```python
from build123d import *

# Parameters (mm, degrees)
F0_R      = 8.001
F0_R_2    = 5.08
F1_DEPTH  = 69.342
F2_R      = 8.001
F2_R_2    = 5.08
F3_ANGLE  = 90
F4_R      = 8.001
F4_R_2    = 5.08
F5_DEPTH  = 76.2
F6_R      = 8.001
F6_R_2    = 5.08
F7_ANGLE  = 30
F8_R      = 8.001
F8_R_2    = 5.08
F9_DEPTH  = 15.24
F10_R     = 8.001
F10_R_2   = 5.08
F11_ANGLE = 30
F12_R     = 8.001
F12_R_2   = 5.08
F13_DEPTH = 50.8


with BuildPart() as f1:
    # F0 (on Front) → F1 (new body)
    with BuildSketch(Plane.XZ):
        Circle(F0_R)
        Circle(F0_R_2, mode=Mode.SUBTRACT)
    extrude(amount=F1_DEPTH)

    # F2 (on face) → F3 (revolve)
    with BuildSketch(Plane.XZ.offset(69.342)):
        Circle(F2_R)
        Circle(F2_R_2, mode=Mode.SUBTRACT)
    revolve(axis=Axis((19.05, -69.342, 0.0863848254), (0, 0, 1)), revolution_arc=F3_ANGLE)

    # F4 (on face) → F5 (join)
    with BuildSketch(Plane.YZ.offset(19.05)):
        with Locations((-88.392, 0)):
            Circle(F4_R)
        with Locations((-88.392, 0)):
            Circle(F4_R_2, mode=Mode.SUBTRACT)
    extrude(amount=F5_DEPTH)

    # F6 (on face) → F7 (revolve)
    with BuildSketch(Plane.YZ.offset(95.25)):
        with Locations((-88.392, 0)):
            Circle(F6_R)
        with Locations((-88.392, 0)):
            Circle(F6_R_2, mode=Mode.SUBTRACT)
    revolve(axis=Axis((95.25, -87.3048111362, -19.05), (0, 1, 0)), revolution_arc=F7_ANGLE)

    # F8 (on face) → F9 (join)
    with BuildSketch(Plane(origin=(79.686391971, 0, -46.0069598552), x_dir=(0, 1, 0), z_dir=(0.8660254038, 0, -0.5))):
        with Locations((-88.392, 50.1772160579)):
            Circle(F8_R)
        with Locations((-88.392, 50.1772160579)):
            Circle(F8_R_2, mode=Mode.SUBTRACT)
    extrude(amount=F9_DEPTH)

    # F10 (on face) → F11 (revolve)
    with BuildSketch(Plane(origin=(92.8846191247, 0, -53.6269598552), x_dir=(0, 1, 0), z_dir=(0.8660254038, 0, -0.5))):
        with Locations((-88.392, 50.1772160579)):
            Circle(F10_R)
        with Locations((-88.392, 50.1772160579)):
            Circle(F10_R_2, mode=Mode.SUBTRACT)
    revolve(axis=Axis((127.4982271537, -88.2504015727, 6.3255678842), (0, -1, 0)), revolution_arc=F11_ANGLE)

    # F12 (on face) → F13 (join)
    with BuildSketch(Plane.YZ.offset(127.4982271537)):
        with Locations((-88.392, -12.7244321158)):
            Circle(F12_R)
        with Locations((-88.392, -12.7244321158)):
            Circle(F12_R_2, mode=Mode.SUBTRACT)
    extrude(amount=F13_DEPTH)


solid = f1.part
```
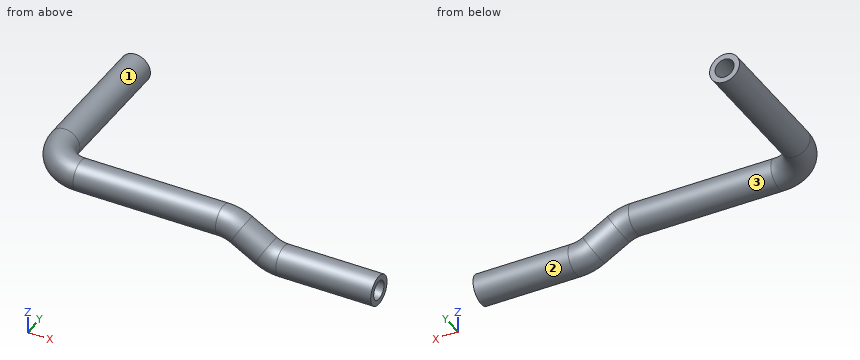
Check sheet for the modelled part. Datum: model origin and axes. Units: mm. Face numbers are marked on the shaded views. Give positions to 0.01 mm unless a question says otherwise; leave off trailing zeros. Order: outer loops, then holes, each group sorted by start corner. A loop starts at its lowest first (then second) coordinate and runs counter-clockwise, first axis right, second up. Notation, with made-up numbers: M 32,43.5 L 49,43.5 A28 cw 49,72.5 Z; hole C -36.75,7.5 d1. An arc over 180 degrees is marked long. Answer in a Markdown table with one row per item. Add a question column.
Q1. Sectioned sample at A-A, the plane x = 77. Record the boundary of the cut face in (y, z).
Q2. Gauge pin test, flat ends, axial feed: pin 1 Ø6 at (y, z) = (-20, 5) entering from +X; pin 2 Ø12 at (y, z) = (-46, -13) entering from -X; pin 3 Ø13 at (y, z) = (-88.39, -12.72) entering from -X. Record the tip position at first contact, or that the pin passes through.
Q3. Release check for a two-part mould opening along X. For the marked faces 1, 2 and 3 record: released by +X, released by -X, zero draft, split by the parting line, or undercut.
Q4. Sectioned sample at B-B, the plane y = -40.5. Record the boundary of the cut face in (x, z).
Q5. Thickness scan on L1, parallel to Z at x = 0, y = -38.5; L2, parallel to Y at x = 16.5, z = -0.5; L3, parallel to X at y = -33, z = -6.25. Record the ranges inside material, lowest first.
Verdict:
| question | item | result |
|---|---|---|
| 1 | outline | C -88.39,0 d16; hole C -88.39,0 d10.16 |
| 2 | pin 1 | x = 7.75 |
| 2 | pin 2 | x = -3.88 |
| 2 | pin 3 | x = 2.51 |
| 3 | face 1 | split by the parting line |
| 3 | face 2 | zero draft |
| 3 | face 3 | undercut |
| 4 | outline | C 0,0 d16; hole C 0,0 d10.16 |
| 5 | L1 | -8 to -5.08, 5.08 to 8 |
| 5 | L2 | -96.26 to -93.31, -83.1 to -80.11 |
| 5 | L3 | -5 to 5 |
